Job drawing, mm, ordinate dimensions from the low corner. One solid piece. A direction names the side the tool comes from. Round coordinates to 2 decimals unless told otherwise and drop trailing zeros. Order: outer loops, then holes, each group sorted by start corner. A loop starts at its lowest first (then second) coordinate and runs counter-clockwise, first axis right, second up. Notation, with made-up numbers: (37.5, -4.75) - (79.5, -4.75) arc R7 cw to (79.5, 8.25) - close; hole circle Ø2 at (29, 84.5). An arc over 180 degrees is marked (long way). Use one line per item in the form item = value. Start each with the question number.
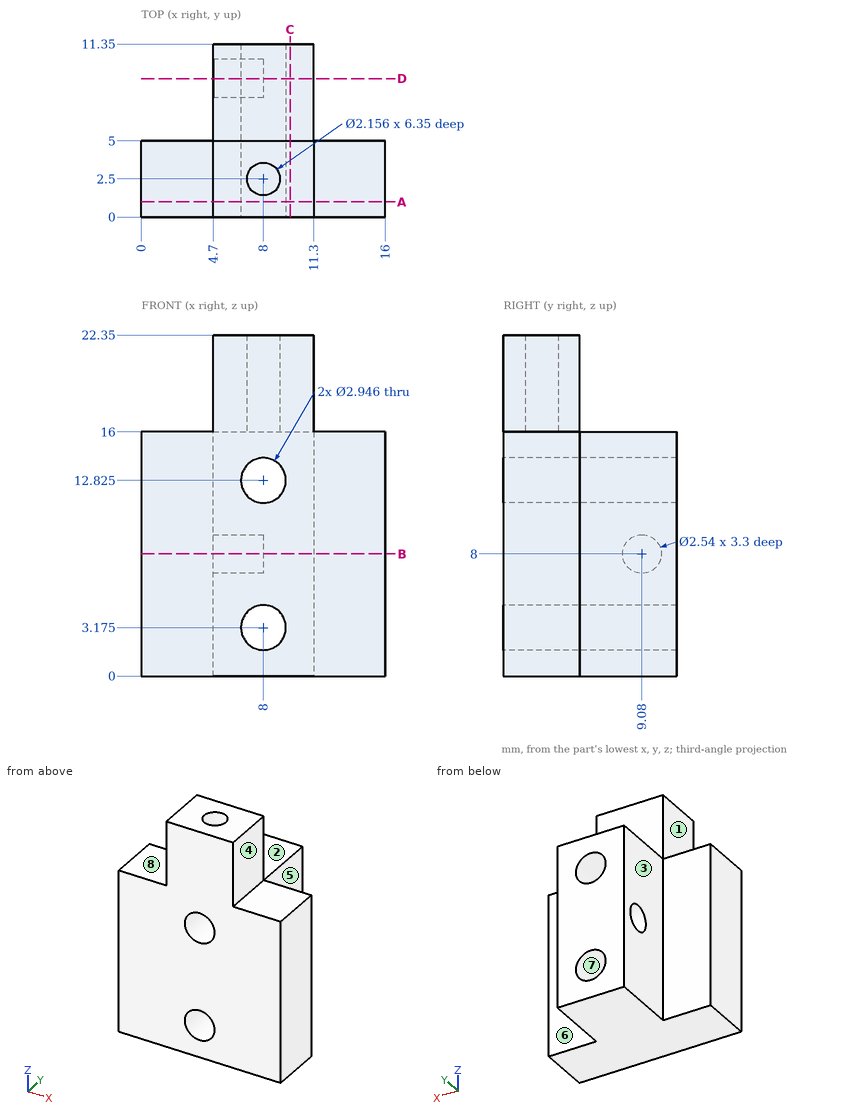
(1) Slice it at D-D (y = 9.08). Give the cut face in (x, z) (1 decimal).
(2) Mould opens along Z. For the marked faces 6, 7 and 8 say: pulls with the +Z half, pulls with the -Z half, needs draft (parallel to the pull), parting line crosses it, or undercut.
(3) Slice it at A-A (y = 1). Give the number of separate pieces and of enclosed holes in the cut face, and give its area (3 significant figures).
(4) Flat gauge pins, fed straight in: P1, Ø2, axis at y = 9, z = 8, coming from the -X side; P2, Ø4, axis at y = 2.5, z = 18.5, coming from the -X side; P3, Ø5.5, axis at y = 3, z = 20.5, coming from the +X side; P4, Ø2.5, axis at x = 8, z = 12.825, coming from the -Y side. Where does each tip first touch, or does it go through?
(5) Wall check: line 1 (Z direction, x = 8, y = 7.5); line 2 (Y direction, x = 8, z = 18.5); line 3 (Y direction, x = 7.35, z = 8). Give the ranges that are in metal, low to high. Write a range as [from, to].
(6) Slice it at B-B (z = 8). Give the cut face in (x, y).
(7) Slice it at C-C (x = 9.75). Give the cut face in (y, z).
(8) Which spindle directions (+Z, -Z, +X, -X, +Y, -Y) get a long thin tool onto all of the face, cutting with end or side? Do the marked faces 1, 2, 3, 4 and 5. Say none if no direction does.
Results list:
q1.outline = (4.7, 0) - (11.3, 0) - (11.3, 16) - (4.7, 16) - (4.7, 9.3) - (8, 9.3) - (8, 6.7) - (4.7, 6.7) - close; hole circle Ø2.9 at (8, 3.2); hole circle Ø2.9 at (8, 12.8)
q2.face_6 = needs draft
q2.face_7 = undercut
q2.face_8 = pulls with the +Z half
q3.separate_pieces = 1
q3.enclosed_holes = 2
q3.area = 284 mm²
q4.P1 = 8
q4.P2 = 4.7
q4.P3 = 11.3
q4.P4 = through
q5.line_1 = [0, 1.7], [4.65, 11.35], [14.3, 16]
q5.line_2 = [0, 1.42], [3.58, 5]
q5.line_3 = [0, 7.81], [10.35, 11.35]
q6.outline = (0, 0) - (16, 0) - (16, 5) - (11.3, 5) - (11.3, 11.35) - (4.7, 11.35) - (4.7, 10.35) - (8, 10.35) - (8, 7.81) - (4.7, 7.81) - (4.7, 5) - (0, 5) - close
q7.outline = (0, 0) - (11.35, 0) - (11.35, 16) - (5, 16) - (5, 22.35) - (0, 22.35) - close
q8.face_1 = +Z, -X, +Y, -Y
q8.face_2 = +Z, +X, -X, +Y
q8.face_3 = +Z, -Z, -X, +Y
q8.face_4 = +Z, +X, +Y, -Y
q8.face_5 = +Z, -Z, +X, +Y
